Can you work these out from the model? Positions are in its coordinate system, mm. A direction names the side the tool comes from. Give positions to 0.01 mm unless a question says otherwise; leave off trailing zeros. Order: outer loops, then holes, each group sorted by start corner. A loop starts at its lowest first (then second) coordinate and runs counter-clockwise, first axis right, second up. Notation, with made-up numbers: (59.25, 39) - (104.25, 39) arc R26 cw to (104.25, 71) - close; hole circle Ø8 at (-28.75, 11.5). An arc over 180 degrees is marked (long way). Answer as a JSON object with one key per item and string values.
```python
from build123d import *

# Parameters (mm, degrees)
SKETCH1_W                = 40
SKETCH1_H                = 11
BOSS_EXTRUDE1_DEPTH      = 19.5
SKETCH2_W                = 70
SKETCH2_H                = 11
BOSS_EXTRUDE2_DEPTH      = 10
SKETCH3_W                = 70
SKETCH3_H                = 20
SKETCH3_W_2              = 40
SKETCH3_H_2              = 19.5
BOSS_EXTRUDE4_DEPTH      = 3
SKETCH4_W                = 70
SKETCH4_H                = 30
SKETCH4_W_2              = 40
SKETCH4_H_2              = 19.5
BOSS_EXTRUDE5_DEPTH      = 3
SKETCH5_R                = 3.264523149
CUT_EXTRUDE1_DEPTH       = 50.132473986
BOSS_EXTRUDE6_DEPTH      = 3
BOSS_EXTRUDE6_DEPTH_BACK = 3
SKETCH6_W                = 40
SKETCH6_H                = 19.5
SKETCH6_H_2              = 39
SKETCH6_R                = 9
FILLET1_R                = 5
FILLET2_R                = 10


with BuildPart() as part:
    # Sketch1 → Boss-Extrude1 (new body)
    with BuildSketch(Plane.XY):
        Rectangle(SKETCH1_W, SKETCH1_H)
    extrude(amount=BOSS_EXTRUDE1_DEPTH)

    # Sketch2 → Boss-Extrude2 (add)
    with BuildSketch(Plane(origin=(0, 0, 0), x_dir=(-1, 0, 0), z_dir=(0, 0, -1))):
        Rectangle(SKETCH2_W, SKETCH2_H)
    extrude(amount=BOSS_EXTRUDE2_DEPTH)

    # Sketch3 → Boss-Extrude4 (add)
    with BuildSketch(Plane(origin=(0, 5.5, 0), x_dir=(1, 0, 0), z_dir=(0, 1, 0))):
        with Locations((0, 20)):
            Rectangle(SKETCH3_W, SKETCH3_H)
        Polygon((-35, 10), (-35, 0), (-20, 0), (20, 0), (35, 0), (35, 10), align=None)
        with Locations((0, -9.75)):
            Rectangle(SKETCH3_W_2, SKETCH3_H_2)
    extrude(amount=BOSS_EXTRUDE4_DEPTH)

    # Sketch4 → Boss-Extrude5 (add)
    with BuildSketch(Plane.XZ.offset(5.5)):
        with Locations((0, -15)):
            Rectangle(SKETCH4_W, SKETCH4_H)
        with Locations((0, 9.75)):
            Rectangle(SKETCH4_W_2, SKETCH4_H_2)
    extrude(amount=BOSS_EXTRUDE5_DEPTH)

    # Sketch5 → Cut-Extrude1 (cut, through all)
    with BuildSketch(Plane.XZ.offset(8.5)):
        with Locations(Location((-20, -20, 0), (0, 0, 270))):
            Circle(SKETCH5_R)
        with Locations(Location((20, -20, 0), (0, 0, 270))):
            Circle(SKETCH5_R)
    extrude(amount=-CUT_EXTRUDE1_DEPTH, mode=Mode.SUBTRACT)

    # Sketch6 → Boss-Extrude6 (add, two sides: drawn at the far end of the back side and taken through both)
    # profile 1 of 3: a face of its own
    with BuildSketch(Plane(origin=(0, 8.5, 0), x_dir=(1, 0, 0), z_dir=(0, 1, 0)).offset(-BOSS_EXTRUDE6_DEPTH_BACK)):
        Polygon((-20, 0), (20, 0), (35, 0), (35, 8.588079042), (-35, 8.588079042), (-35, 0), align=None)
    # profile 2 of 3: a face of its own
    with BuildSketch(Plane(origin=(0, 8.5, 0), x_dir=(1, 0, 0), z_dir=(0, 1, 0)).offset(-BOSS_EXTRUDE6_DEPTH_BACK)):
        with Locations((0, -9.75)):
            Rectangle(SKETCH6_W, SKETCH6_H)
    # profile 3 of 3: a face of its own
    with BuildSketch(Plane(origin=(0, 8.5, 0), x_dir=(1, 0, 0), z_dir=(0, 1, 0)).offset(-BOSS_EXTRUDE6_DEPTH_BACK)):
        with Locations((0, -39)):
            Rectangle(SKETCH6_W, SKETCH6_H_2)
        with Locations(Location((0, -40, 0), (0, 0, 270))):
            Circle(SKETCH6_R, mode=Mode.SUBTRACT)
    extrude(amount=BOSS_EXTRUDE6_DEPTH + BOSS_EXTRUDE6_DEPTH_BACK)

    # Fillet1
    # the kernel refuses this fillet: 5 mm, written as the material it adds along each edge
    with BuildSketch(Plane(origin=(-35, 8.5, -8.588079042), x_dir=(0, 0, -1), z_dir=(1, 0, 0))) as fillet1_piece_1:
        with BuildLine():
            CenterArc((4.582575695, 5), FILLET1_R, 203.578178478, 66.421821522)
            Line((0, 3), (-0.091651514, 2.96))
            ThreePointArc((-0.091651514, 2.96), (-0.1, 1.5), (-0.1, 0))
            Line((-0.1, 0), (0, -0.1))
            Line((0, -0.1), (4.582575695, -0.1))
            Line((4.582575695, -0.1), (4.582575695, 0))
        make_face()
    extrude(amount=70)

    # Fillet2
    fillet2_edges = [part.edges().sort_by_distance(p)[0] for p in [
        (-20, 1.5, 0),
        (20, 1.5, 0),
    ]]
    fillet(fillet2_edges, radius=FILLET2_R)


solid = part.part
```
Q1. I need wall thicknesses on L1, parallel to X at y = 7.3, z = -20; L2, parallel to Y at x = 8, z = -19; L3, parallel to X at y = 9.4, z = 40. Which ranges of each line are inside material? Lowest first, please.
Recorded:
{"L1": "x = -35 to -23.26, -16.74 to 16.74, 23.26 to 35", "L2": "y = -8.5 to -5.5, 5.5 to 8.5", "L3": "x = -20 to -9, 9 to 20"}
Q2. If we section it at C-C, the plane y = 3.25: Please give me the cut outline in (x, z), then the cut area to 3 significant figures.
Recorded:
{"outline": "(-35, -10) - (35, -10) - (35, 0) - (30, 0) arc R10 cw to (20, 10) - (20, 19.5) - (-20, 19.5) - (-20, 10) arc R10 cw to (-30, 0) - (-35, 0) - close", "area": "1,520 mm^2"}
Q3. If we section it at A-A, the plane x = 0: Please give me the cut outline in (y, z), then the cut area to 3 significant figures.
Recorded:
{"outline": "(-8.5, -30) - (-5.5, -30) - (-5.5, -10) - (5.5, -10) - (5.5, -30) - (8.5, -30) - (8.5, -13.17) arc R5 cw to (11.5, -8.59) - (11.5, 31) - (5.5, 31) - (5.5, 19.5) - (-8.5, 19.5) - close; (5.5, 49) - (11.5, 49) - (11.5, 58.5) - (5.5, 58.5) - close", "area": "836 mm^2"}
Q4. I'm going to push flat-ended pins straight in: pin 1 Ø22 at (x, z) = (2, -16.5) entering from +Y; pin 2 Ø5.5 at (x, y) = (32, -3) entering from +Z; pin 3 Ø5.5 at (x, y) = (-10.5, -1.5) entering from -Z; pin 4 Ø2 at (x, y) = (4, 1) entering from +Z. Where does each tip first touch, or does it pass through?
Recorded:
{"pin 1": "stops at y = 11.5", "pin 2": "stops at z = 0.03", "pin 3": "stops at z = -10", "pin 4": "stops at z = 19.5"}
Q5. We'd pull the mould along X, two halves only. Please class faces 1 (the face through (22.85, 1.36, 3.01)), 2 (the face through (18.75, 6.979, -23.016)), 3 (the face through (-23.01, 1.64, 2.85)), 4 (the face through (0, -5.5, -20)): released by +X, released by -X, zero draft, split by the parting line, or undercut.
Recorded:
{"face 1": "released by +X", "face 2": "undercut", "face 3": "released by -X", "face 4": "zero draft"}
Q6. If we section it at D-D, the plane z = 39: Please give me the cut outline in (x, y), then the cut area to 3 significant figures.
Recorded:
{"outline": "(-20, 5.5) - (-8.94, 5.5) - (-8.94, 11.5) - (-20, 11.5) - close; (8.94, 5.5) - (20, 5.5) - (20, 11.5) - (8.94, 11.5) - close", "area": "133 mm^2"}
Q7. Which directions (+Z, -Z, +X, -X, +Y, -Y) give clear straight access to the entire face, cutting with the end or side of a thin tool? Please do faces 5 (the face through (0, 0, -10)), 6 (the face through (0, -1, 19.5)), 7 (the face through (20, 6, 29)), 8 (the face through (-20, 6, 29)).
Recorded:
{"face 5": "-Z, +X, -X", "face 6": "+Z, +X, -X, -Y", "face 7": "+Z, +X, +Y, -Y", "face 8": "+Z, -X, +Y, -Y"}
Q8. If we section it at B-B, the plane z = -20: Please give me the cut outline in (x, y), then the cut area to 3 significant figures.
Recorded:
{"outline": "(-35, -8.5) - (-23.26, -8.5) - (-23.26, -5.5) - (-35, -5.5) - close; (-35, 5.5) - (-23.26, 5.5) - (-23.26, 8.5) - (-35, 8.5) - close; (-16.74, -8.5) - (16.74, -8.5) - (16.74, -5.5) - (-16.74, -5.5) - close; (-16.74, 5.5) - (16.74, 5.5) - (16.74, 8.5) - (-16.74, 8.5) - close; (23.26, -8.5) - (35, -8.5) - (35, -5.5) - (23.26, -5.5) - close; (23.26, 5.5) - (35, 5.5) - (35, 8.5) - (23.26, 8.5) - close", "area": "342 mm^2"}
